```python
from build123d import *

# Parameters (mm, degrees)
F0_W      = 1000
F0_H      = 740
F1_DEPTH  = 500
F3_DEPTH  = 400
F4_R      = 80
F5_DEPTH  = 100.001
F7_DEPTH  = 400
F8_W      = 500
F8_H      = 130
F9_DEPTH  = 220
F10_W     = 500
F10_H     = 130
F11_DEPTH = 220
F12_W     = 500
F12_H     = 610
F13_DEPTH = 220
F15_DEPTH = 500.001
F17_DEPTH = 420
F18_W     = 500
F18_H     = 610
F19_DEPTH = 220
F21_DEPTH = 500.001
F23_DEPTH = 420
F24_R     = 80
F25_DEPTH = 50
F26_R     = 40


with BuildPart() as f1:
    # F0 (on Front) → F1 (new body)
    with BuildSketch(Plane.XZ):
        Rectangle(F0_W, F0_H)
    extrude(amount=F1_DEPTH)

    # F2 (on face) → F3 (cut)
    with BuildSketch(Plane.XZ.offset(500)):
        with BuildLine():
            ThreePointArc((320, 130), (308.284271, 158.284271), (280, 170))
            Line((280, 170), (-280, 170))
            ThreePointArc((-280, 170), (-308.284271, 158.284271), (-320, 130))
            Line((-320, 130), (-320, -180))
            ThreePointArc((-320, -180), (-308.284271, -208.284271), (-280, -220))
            Line((-280, -220), (280, -220))
            ThreePointArc((280, -220), (308.284271, -208.284271), (320, -180))
            Line((320, -180), (320, 130))
        make_face()
    extrude(amount=-F3_DEPTH, mode=Mode.SUBTRACT)

    # F4 (on face) → F5 (cut, through all)
    with BuildSketch(Plane.XZ.offset(100)):
        with Locations((0, -25)):
            Circle(F4_R)
    extrude(amount=-F5_DEPTH, mode=Mode.SUBTRACT)

    # F6 (on face) → F7 (cut)
    with BuildSketch(Plane.XZ.offset(500)):
        with BuildLine():
            Line((450, 260), (450, 520))
            Line((450, 520), (-450, 520))
            Line((-450, 520), (-450, 260))
            ThreePointArc((-450, 260), (-438.284271, 231.715729), (-410, 220))
            Line((-410, 220), (410, 220))
            ThreePointArc((410, 220), (438.284271, 231.715729), (450, 260))
        make_face()
    extrude(amount=-F7_DEPTH, mode=Mode.SUBTRACT)

    # F8 (on face) → F9 (join)
    with BuildSketch(Plane.YZ.offset(500)):
        with Locations((-250, -305)):
            Rectangle(F8_W, F8_H)
    extrude(amount=F9_DEPTH)

    # F10 (on face) → F11 (join)
    with BuildSketch(Plane(origin=(-500, 0, 0), x_dir=(0, -1, 0), z_dir=(-1, 0, 0))):
        with Locations((250, -305)):
            Rectangle(F10_W, F10_H)
    extrude(amount=F11_DEPTH)

    # F12 (on face) → F13 (join)
    with BuildSketch(Plane(origin=(-500, 0, 0), x_dir=(0, -1, 0), z_dir=(-1, 0, 0))):
        with Locations((250, 65)):
            Rectangle(F12_W, F12_H)
    extrude(amount=F13_DEPTH)

    # F14 (on face) → F15 (cut, through all)
    with BuildSketch(Plane.XZ.offset(500)):
        Polygon((-720, 370), (-720, 0), (-500, 370), align=None)
    extrude(amount=-F15_DEPTH, mode=Mode.SUBTRACT)

    # F16 (on face) → F17 (cut)
    with BuildSketch(Plane.XZ.offset(500)):
        Polygon((-500, -240), (-500, 370), (-720, 0), (-720, -240), align=None)
    extrude(amount=-F17_DEPTH, mode=Mode.SUBTRACT)

    # F18 (on face) → F19 (join)
    with BuildSketch(Plane.YZ.offset(500)):
        with Locations((-250, 65)):
            Rectangle(F18_W, F18_H)
    extrude(amount=F19_DEPTH)

    # F20 (on face) → F21 (cut, through all)
    with BuildSketch(Plane.XZ.offset(500)):
        Polygon((720, 370), (500, 370), (720, 0), align=None)
    extrude(amount=-F21_DEPTH, mode=Mode.SUBTRACT)

    # F22 (on face) → F23 (cut)
    with BuildSketch(Plane.XZ.offset(500)):
        Polygon((720, 0), (500, 370), (500, -240), (720, -240), align=None)
    extrude(amount=-F23_DEPTH, mode=Mode.SUBTRACT)

    # F24 (on face) → F25 (cut)
    with BuildSketch(Plane.XY.offset(220)):
        with Locations((0, -300)):
            Circle(F24_R)
    extrude(amount=-F25_DEPTH, mode=Mode.SUBTRACT)

    # F26
    f26_edges = [f1.edges().sort_by_distance(p)[0] for p in [
        (-500, -290, -240),
        (500, -290, -240),
    ]]
    fillet(f26_edges, radius=F26_R)


solid = f1.part
```
Verification items for the finished model (mm, model axes). A direction names the side the tool comes from. Coordinates: 2 decimals unless noted, no trailing zeros. Write each loop counter-clockwise with the first axis right and the second up, starting at its lowest first coordinate (ties: lowest second). Pieces come first, ordered by that corner, then holes. Notation, with made-up numbers: (47.5, 12) - (75.5, 12) arc R37 ccw to (75.5, 48) - close; hole circle Ø1 at (-21.75, -25). An arc over 180 degrees is marked (long way). Write item = value, one per line.
Q1. Cross-section at C-C (z = -61). Enter the section's corners in (x, y).
Answer:
outline = (-720, -80) - (-500, -80) - (-500, -500) - (-320, -500) - (-320, -100) - (-71.44, -100) - (-71.44, 0) - (-720, 0) - close; (71.44, -100) - (320, -100) - (320, -500) - (500, -500) - (500, -80) - (720, -80) - (720, 0) - (71.44, 0) - close
Q2. Access from +Z, -Z, +X, -X, +Y, -Y to the whole of each face (thin tool, end or side, straight path). Record for faces 1 (the face through (511.406, -287.06, -227.972)), 2 (the face through (-587, -80, 1)), 3 (the face through (66, -347, 170)).
Answer:
face_1 = +Z, +X, -Y
face_2 = +Z, -X, -Y
face_3 = -Y
Q3. Cross-section at B-B (y = -168). Enter the section's corners in (x, z), plus the area to 3 significant figures.
Answer:
outline = (-720, -370) - (720, -370) - (720, -240) - (540, -240) arc R40 cw to (500, -200) - (500, 370) - (450, 370) - (450, 260) arc R40 cw to (410, 220) - (-410, 220) arc R40 cw to (-450, 260) - (-450, 370) - (-500, 370) - (-500, -200) arc R40 cw to (-540, -240) - (-720, -240) - close; hole (-320, -180) arc R40 ccw to (-280, -220) - (280, -220) arc R40 ccw to (320, -180) - (320, 130) arc R40 ccw to (280, 170) - (-280, 170) arc R40 ccw to (-320, 130) - close
area = 415,000 mm²
Q4. Material ranges on L1, parallel to X at y = -359.5, z = 264.5; L2, parallel to Z at x = 190, y = -251; L3, parallel to X at y = -150, z = -83, recorded low to high. Write a range as from..to.
Answer:
L1 = -500..-450, 450..500
L2 = -370..-220, 170..220
L3 = -500..-320, 320..500
Q5. Go/stop test with flat-tipped pins: pin 1 Ø8 at (y, z) = (-381, 283) entering from -X; pin 2 Ø4 at (y, z) = (-99.5, -231) entering from +X; pin 3 Ø4 at (x, y) = (399.5, -256) entering from +Z. Record where each tip stops, or that it passes through.
Answer:
pin_1 = -500
pin_2 = 517.39
pin_3 = 220
Q6. Cross-section at A-A (x = 0). Enter the section's corners in (y, z), plus the area to 3 significant figures.
Answer:
outline = (-500, -370) - (0, -370) - (0, -105) - (-100, -105) - (-100, -220) - (-500, -220) - close; (-500, 170) - (-380, 170) - (-380, 220) - (-500, 220) - close; (-220, 170) - (-100, 170) - (-100, 55) - (0, 55) - (0, 370) - (-100, 370) - (-100, 220) - (-220, 220) - close
area = 130,000 mm²
Q7. Mould release check, pull along Z, two halves, no side actions. Record for faces 4 (the face through (-512.028, -287.06, -228.594)), 5 (the face through (-10, -500, -252)), 6 (the face through (-320, -303, -23)): released by +Z, released by -Z, zero draft, split by the parting line, or undercut.
Answer:
face_4 = released by +Z
face_5 = zero draft
face_6 = undercut
Q8. Cross-section at D-D (x = 145.5). Enter the section's corners in (y, z), plus the area to 3 significant figures.
Answer:
outline = (-500, -370) - (0, -370) - (0, 370) - (-100, 370) - (-100, 220) - (-500, 220) - (-500, 170) - (-100, 170) - (-100, -220) - (-500, -220) - close
area = 154,000 mm²
